Autodesk Inventor part; units mm, degrees
ref_plane "YZ Plane" through (0, 0, 0) normal (1, 0, 0) x (0, 1, 0)
ref_plane "XZ Plane" through (0, 0, 0) normal (0, 1, 0) x (-1, 0, 0)
ref_plane "XY Plane" through (0, 0, 0) normal (0, 0, 1) x (1, 0, 0)
sketch "Sketch1" plane through (0, 0, 0) normal (0, 1, 0) x (-1, 0, 0)
  circle A0 centre (0, 0) radius 2.45
  dimension "d0" = 4.9
extrude "Extrusion1" add sketch "Sketch1" along normal blind 50
sketch "Sketch2" plane through (0, 50, 0) normal (0, 1, 0) x (1, 0, 0)
  circle A0 centre (0, 0) radius 3.5
  dimension "d3" = 7
extrude "Extrusion2" add sketch "Sketch2" along normal blind 2
thread "Thread1"
sketch "Sketch3" plane through (0, 52, 0) normal (0, 1, 0) x (1, 0, 0)
  line L0 (0.866, 1.5) -> (1.7321, 0)
  line L1 (1.7321, 0) -> (0.866, -1.5)
  line L2 (0.866, -1.5) -> (-0.866, -1.5)
  line L3 (-0.866, -1.5) -> (-1.7321, 0)
  line L4 (-1.7321, 0) -> (-0.866, 1.5)
  line L5 (-0.866, 1.5) -> (0.866, 1.5)
  point P0 (0, 0)
  point P1 (0, 0)
  dimension "d8" = 3
extrude "Extrusion3" cut sketch "Sketch3" against normal blind 1
equation "\"BendRadius\" = Thickness"
equation "\"BendReliefWidth\" = Thickness"
equation "\"BendReliefDepth\" = 0.5 * Thickness"
equation "\"CornerReliefSize\" = 4 * Thickness"
equation "\"MinimumRemnant\" = 2 * Thickness"
equation "\"TransitionRadius\" = BendRadius"
equation "\"JacobiRadiusSize\" = BendRadius"
equation "\"GapSize\" = Thickness"
properties part number "perno_simple"
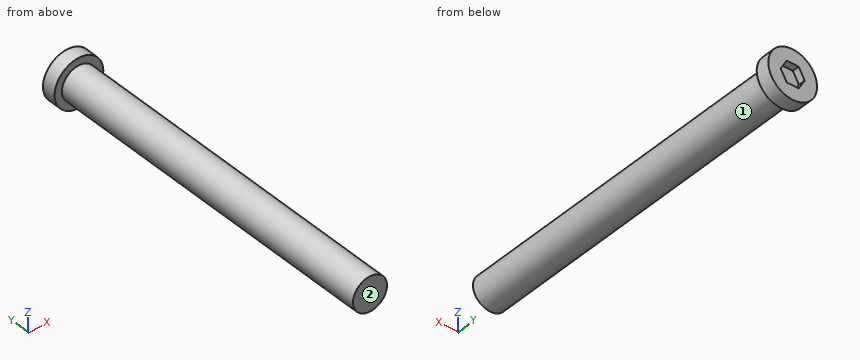
Build history of the part. All positions in model axes, mm. Face numbers are marked on the shaded views. A direction names the side the tool comes from. Coordinates: 2 decimals unless noted, no trailing zeros. Write each loop counter-clockwise with the first axis right and the second up, starting at its lowest first coordinate (ties: lowest second). Pieces come first, ordered by that corner, then holes.
(1) Cut at A-A on x = 0. List the corners of the cut face in (y, z), and give its area (3 significant figures).
(2) Cut at C-C on y = 40.5. List the corners of the cut face in (x, z).
(3) Pin check, flat tips, straight feed: pin 1 Ø3 at (y, z) = (38.5, 2.5) entering from -X; pin 2 Ø1.5 at (y, z) = (16.5, 1.5) entering from +X. Stop position of each tip, or through.
(4) Drill centre lines: line 1 (Y direction, x = -0.5, z = 1); line 2 (Y direction, x = -0.25, z = 3); line 3 (X direction, y = 34.5, z = -1). Where is each one in solid material? Low to high.
(5) 3-axis set-ups, long thin cutter, end or side, ignore diameter. For the marked faces 1 and 2: which of +Z, -Z, +X, -X, +Y, -Y reach the whole face in a straight line?
(6) Cut at B-B on z = 0.5. List the corners of the cut face in (x, y), and give its area (3 significant figures).
Working result:
1. outline: (0, -2.45) - (50, -2.45) - (50, -3.5) - (52, -3.5) - (52, -1.5) - (51, -1.5) - (51, 1.5) - (52, 1.5) - (52, 3.5) - (50, 3.5) - (50, 2.45) - (0, 2.45) - close
1. area: 256 mm2
2. outline: circle Ø4.9 at (0, 0)
3. pin 1: stops at x = -2.24
3. pin 2: stops at x = 2.33
4. line 1: y = 0 to 51
4. line 2: y = 50 to 52
4. line 3: x = -2.24 to 2.24
5. face 1: -Y
5. face 2: +Z, -Z, +X, -X, -Y
6. outline: (-3.46, 50) - (-2.4, 50) - (-2.4, 0) - (2.4, 0) - (2.4, 50) - (3.46, 50) - (3.46, 52) - (1.44, 52) - (1.44, 51) - (-1.44, 51) - (-1.44, 52) - (-3.46, 52) - close
6. area: 251 mm2
